Input: part model. Units: mm. Frame: model coordinates. A direction names the side the tool comes from. Coordinates: 2 decimals unless noted, no trailing zeros. Write each loop counter-clockwise with the first axis right and the second up, starting at its lowest first coordinate (ties: lowest second). Pieces come first, ordered by that corner, then holes. Notation, with made-up numbers: M 10.5,-8 L 23.5,-8 A35 ccw 23.5,27 Z; hole C -1,6.25 d3. An arc over 180 degrees is marked long. Use one line per item in the form item = value.
from build123d import *

# Parameters (mm, degrees)
ESQUISSE1_W             = 190
ESQUISSE1_H             = 20
BOSS_EXTRU_1_DEPTH      = 10
ESQUISSE2_W             = 6
ESQUISSE2_H             = 20
ENL_V_MAT_EXTRU_1_DEPTH = 6
ESQUISSE3_R             = 1.5
ENL_V_MAT_EXTRU_2_DEPTH = 6


with BuildPart() as part:
    # Esquisse1 → Boss.-Extru.1 (new body)
    with BuildSketch(Plane.XY):
        Rectangle(ESQUISSE1_W, ESQUISSE1_H)
    extrude(amount=BOSS_EXTRU_1_DEPTH)

    # Esquisse2 → Enlèv. mat.-Extru.1 (cut)
    with BuildSketch(Plane.XY.offset(10)):
        with Locations((-92, 0)):
            Rectangle(ESQUISSE2_W, ESQUISSE2_H)
        with Locations((92, 0)):
            Rectangle(ESQUISSE2_W, ESQUISSE2_H)
    extrude(amount=-ENL_V_MAT_EXTRU_1_DEPTH, mode=Mode.SUBTRACT)

    # Esquisse3 → Enlèv. mat.-Extru.2 (cut)
    with BuildSketch(Plane(origin=(0, 0, 0), x_dir=(-1, 0, 0), z_dir=(0, 0, -1))):
        with Locations((92, 0)):
            Circle(ESQUISSE3_R)
    extrude(amount=-ENL_V_MAT_EXTRU_2_DEPTH, mode=Mode.SUBTRACT)


solid = part.part
(1) Set-up query: faces 5 (the flat face through (92, 0, 4)), 6 (the flat face through (-89, 0, 7)), 7 (the flat face through (-1, 10, 5)). Return all of +Z, -Z, +X, -X, +Y, -Y with unobstructed straight access to the full face (end or side cutting, diameter ignored); none if empty.
Computed:
face_5 = +Z, +X, +Y, -Y
face_6 = +Z, -X, +Y, -Y
face_7 = +Z, -Z, +X, -X, +Y
(2) First-contact query: pin 1 Ø3 at (x, y) = (-92.5, 2) entering from +Z; pin 2 Ø1.8 at (y, z) = (-2.5, 7.5) entering from -X; pin 3 Ø1.8 at (y, z) = (0, 8) entering from +X. Flat tips, straight axial feed; report the tip coordinate or a pass-through.
Computed:
pin_1 = 4
pin_2 = -89
pin_3 = 89
(3) Pull-direction query (X, two-part tool) for faces 1 (the flat face through (-1, -10, 5)), 2 (the flat face through (89, 0, 7)), 3 (the cylindrical face through (-93.43, 0.45, 1.97)), 4 (the flat face through (-95, 0, 2)); classes: pulls with the +X half, pulls with the -X half, needs draft (parallel to the pull), parting line crosses it, or undercut.
Computed:
face_1 = needs draft
face_2 = pulls with the +X half
face_3 = undercut
face_4 = pulls with the -X half
(4) Section query A-A on y = 5.75. Return the cut outline in (x, z), plus the area to 3 significant figures.
Computed:
outline = M -95,0 L 95,0 L 95,4 L 89,4 L 89,10 L -89,10 L -89,4 L -95,4 Z
area = 1,830 mm^2
(5) Line query: probe 1 along Y at (x, z) = (-92, 0.95); probe 2 along X at (y, z) = (5.25, 6.75). Output: solid intervals per line, ascending.
Computed:
probe_1 = -10 to -1.5, 1.5 to 10
probe_2 = -89 to 89
